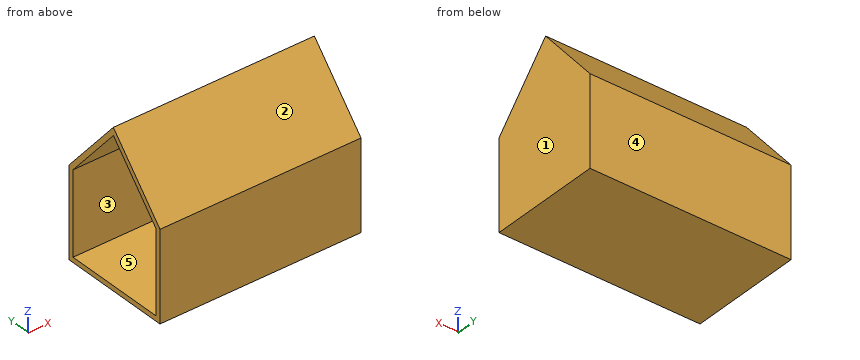
from build123d import *

# Parameters (mm, degrees)
F0_W     = 57.356569916
F0_H     = 45.3068669885
F1_DEPTH = 101.6
F2_T     = -2.54


with BuildPart() as f1:
    # F0 (on Right) → F1 (new body)
    with BuildSketch(Plane.YZ):
        with Locations((-0.7229857147, -5.7838549837)):
            Rectangle(F0_W, F0_H)
        Polygon((0, 49.8857535422), (-29.4012706727, 16.8695785105), (27.9552992433, 16.8695785105), align=None)
    extrude(amount=F1_DEPTH)

    # F2
    f2_openings = [f1.faces().sort_by_distance(p)[0] for p in [
        (0, -0.658626, 3.204954),
    ]]
    offset(amount=F2_T, openings=f2_openings)


solid = f1.part
For this review, take the finished solid that the model builds, in its own axes (mm). Face numbers are marked on the shaded views. A direction names the side the tool comes from. Coordinates: 2 decimals unless noted, no trailing zeros. Write each loop counter-clockwise with the first axis right and the second up, starting at its lowest first coordinate (ties: lowest second). Pieces come first, ordered by that corner, then holes. Notation, with made-up numbers: (40.5, 67.5) -> (91.5, 67.5) arc R7 ccw to (91.5, 79.5) -> close; hole circle Ø11 at (55, 48). An arc over 180 degrees is marked (long way). Write each question's results on one line, items separated by ' | '. Start each with the question number.
1) The part is to be moulded in two halves that separate along Y. For the marked faces 1, 2 and 3, say which applies: +Y half, -Y half, draft (parallel to the pull), parting line (faces both ways), or undercut.
2) Insertion check: pin 1 (2 mm diameter, centred on y = 12.5, z = -5, fed in from -X); pin 2 (5 mm diameter, centred on x = 45, y = -21, fed in from +Z). Each pin has a flat end and moves straight along its axis. Give the tip position at first contact, or say it passes through.
3) For the marked faces 4 and 5, list the 3-axis set-ups (+Z, -Z, +X, -X, +Y, -Y) from which the entire face can be reached by the end or side of a thin tool; tool diameter is ignored.
4) Consider section B-B (z = -11.5). Write out the cut boundary in (x, y), plus the area to 3 significant figures.
5) Wall thickness on L1, parallel to Y at x = 12.5, z = -1.5; L2, parallel to X at y = 11, z = -7; L3, parallel to Z at x = 61, y = -12.5: over which ranges is each line inside the solid? List them lowest first. Write a range as [from, to].
6) Consider section C-C (y = 13.5). Write out the cut boundary in (x, z).
7) Consider section A-A (x = 94.5). Write out the cut boundary in (y, z).
Geometry says:
1) face 1: draft | face 2: -Y half | face 3: undercut
2) pin 1: x = 99.06 | pin 2: z = 29.11
3) face 4: +Z, -Z, +X, -X, +Y | face 5: -X
4) outline: (0, -29.4) -> (101.6, -29.4) -> (101.6, 27.96) -> (0, 27.96) -> (0, 25.42) -> (99.06, 25.42) -> (99.06, -26.86) -> (0, -26.86) -> close | area: 649 mm^2
5) L1: [-29.4, -26.86], [25.42, 27.96] | L2: [99.06, 101.6] | L3: [-28.44, -25.9], [32.03, 35.85]
6) outline: (0, -28.44) -> (101.6, -28.44) -> (101.6, 33.94) -> (0, 33.94) -> (0, 30.01) -> (99.06, 30.01) -> (99.06, -25.9) -> (0, -25.9) -> close
7) outline: (-29.4, -28.44) -> (27.96, -28.44) -> (27.96, 16.87) -> (0, 49.89) -> (-29.4, 16.87) -> close; hole (-26.86, -25.9) -> (25.42, -25.9) -> (25.42, 15.94) -> (-0.05, 46.01) -> (-26.86, 15.9) -> close
